Read the model definition and answer for the solid it produces. Units are mm, in the model's axes. Face numbers are marked on the shaded views. A direction names the side the tool comes from. Give positions to 0.01 mm unless a question says otherwise; leave off trailing zeros. Loops run counter-clockwise (first coordinate to the right, second up) from the corner with the lowest first, then second, coordinate; pieces in that order, holes last. Notation, with made-up numbers: (-38.5, 3) - (-19.5, 3) arc R17 ccw to (-19.5, 26) - close; hole circle Ø4 at (-35.5, 20). An arc over 180 degrees is marked (long way). Use a Markdown table: item, result. Add a question column.
Item 1: For a pull along X with two mould halves and no side action, classify the marked faces 5, 6, 7 and 8 as +X half, -X half, draft (parallel to the pull), parting line (faces both ways), or undercut.
Item 2: A cutting plane is placed at A-A (y = 9). Determine the outline of the cut face in (x, z), plus the area to 3 significant figures.
Item 3: A cutting plane is placed at C-C (x = 0). Determine the outline of the cut face in (y, z).
Item 4: A cutting plane is placed at B-B (z = 6.5). Determine the outline of the cut face in (x, y).
Item 5: Which of the six approach directions +Z, -Z, +X, -X, +Y, -Y give full straight-line access (tool end or side, diameter ignored) to the marked faces 1, 2, 3 and 4?
Item 6: A cutting plane is placed at D-D (x = -4.05). Determine the outline of the cut face in (y, z).
Item 7: Each of these flat-tipped pins is pushed along its axis until it touches: P1, Ø0.6, axis at y = -24.5, z = 0.5, coming from the +X side; P2, Ø1.5, axis at x = -6.5, z = 4.5, coming from the -Y side; P3, Ø1, axis at x = 9, z = 1.5, coming from the +Y side; P4, Ø2.5, axis at x = 4.05, y = 24, coming from the -Z side. Where does it stop, or does it pass through?
Item 8: Consider probe 1 along Y at (x, z) = (4.05, 0.55); probe 2 along Y at (x, z) = (-4.05, 1.05); probe 3 along Y at (x, z) = (0, 4). Determine where each line is inside the solid, lowest interval first. Write a range as [from, to].
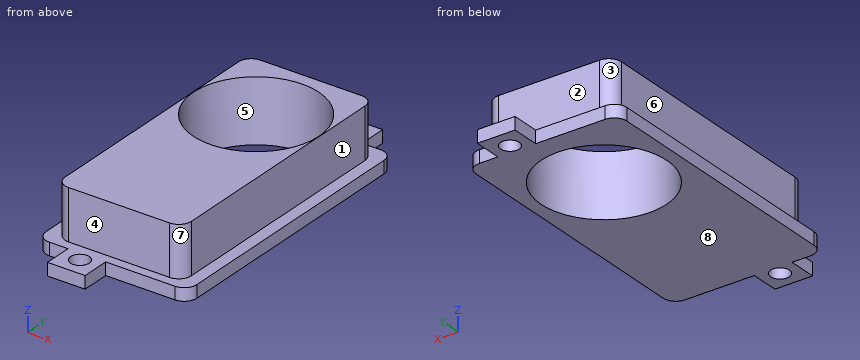
from build123d import *

# Parameters (mm, degrees)
SKETCH1_R           = 1.5
BOSS_EXTRUDE1_DEPTH = 2
FILLET1_R           = 2
SKETCH3_W           = 20.1
SKETCH3_H           = 42
BOSS_EXTRUDE2_DEPTH = 8
FILLET2_R           = 2
SKETCH5_R           = 10
CUT_EXTRUDE3_DEPTH  = 11


with BuildPart() as part:
    # Sketch1 → Boss-Extrude1 (new body)
    with BuildSketch(Plane.XY):
        Polygon((1.05, 22.5), (1.05, 27), (7.05, 27), (7.05, 22.5), (12, 22.5), (12, -22.5), (-1.05, -22.5), (-1.05, -27), (-7.05, -27), (-7.05, -22.5), (-12, -22.5), (-12, 22.5), align=None)
        with Locations((4.05, 24)):
            Circle(SKETCH1_R, mode=Mode.SUBTRACT)
        with Locations((-4.05, -24)):
            Circle(SKETCH1_R, mode=Mode.SUBTRACT)
    extrude(amount=BOSS_EXTRUDE1_DEPTH)

    # Fillet1
    fillet1_edges = [part.edges().sort_by_distance(p)[0] for p in [
        (12, 22.5, 1),
        (12, -22.5, 1),
        (-12, -22.5, 1),
        (-12, 22.5, 1),
    ]]
    fillet(fillet1_edges, radius=FILLET1_R)

    # Sketch3 → Boss-Extrude2 (add)
    with BuildSketch(Plane.XY.offset(2)):
        Rectangle(SKETCH3_W, SKETCH3_H)
    extrude(amount=BOSS_EXTRUDE2_DEPTH)

    # Fillet2
    fillet2_edges = [part.edges().sort_by_distance(p)[0] for p in [
        (-10.05, 21, 6),
        (-10.05, -21, 6),
        (10.05, -21, 6),
        (10.05, 21, 6),
    ]]
    fillet(fillet2_edges, radius=FILLET2_R)

    # Sketch5 → Cut-Extrude3 (cut, through all)
    with BuildSketch(Plane.XY.offset(10)):
        with Locations((0, 9)):
            Circle(SKETCH5_R)
    extrude(amount=-CUT_EXTRUDE3_DEPTH, mode=Mode.SUBTRACT)


solid = part.part
Geometry says:
| question | item | result |
|---|---|---|
| 1 | face 5 | undercut |
| 1 | face 6 | -X half |
| 1 | face 7 | +X half |
| 1 | face 8 | draft |
| 2 | outline | (-12, 0) - (-10, 0) - (-10, 10) - (-10.05, 10) - (-10.05, 2) - (-12, 2) - close; (10, 0) - (12, 0) - (12, 2) - (10.05, 2) - (10.05, 10) - (10, 10) - close |
| 2 | area | 8.80 mm² |
| 3 | outline | (-22.5, 0) - (-1, 0) - (-1, 10) - (-21, 10) - (-21, 2) - (-22.5, 2) - close; (19, 0) - (22.5, 0) - (22.5, 2) - (21, 2) - (21, 10) - (19, 10) - close |
| 4 | outline | (-10.05, -19) arc R2 ccw to (-8.05, -21) - (8.05, -21) arc R2 ccw to (10.05, -19) - (10.05, 19) arc R2 ccw to (8.05, 21) - (-8.05, 21) arc R2 ccw to (-10.05, 19) - close; hole circle Ø20 at (0, 9) |
| 5 | face 1 | +Z, +X, +Y, -Y |
| 5 | face 2 | +Z, +X, -X, +Y |
| 5 | face 3 | +Z, -X, +Y |
| 5 | face 4 | +Z, +X, -X, -Y |
| 6 | outline | (-27, 0) - (-25.5, 0) - (-25.5, 2) - (-27, 2) - close; (-22.5, 0) - (-0.14, 0) - (-0.14, 10) - (-21, 10) - (-21, 2) - (-22.5, 2) - close; (18.14, 0) - (22.5, 0) - (22.5, 2) - (21, 2) - (21, 10) - (18.14, 10) - close |
| 7 | P1 | x = -1.05 |
| 7 | P2 | y = -21 |
| 7 | P3 | y = 22.5 |
| 7 | P4 | through |
| 8 | probe 1 | [-22.5, -0.14], [18.14, 22.5], [25.5, 27] |
| 8 | probe 2 | [-27, -25.5], [-22.5, -0.14], [18.14, 22.5] |
| 8 | probe 3 | [-21, -1], [19, 21] |
